from build123d import *

# Parameters (mm, degrees)
SKETCH_1_W          = 100
SKETCH_1_H          = 110
SKETCH_1_R          = 35
EXTRUDE_1_DEPTH     = 10
SKETCH_2_W          = 6
SKETCH_2_H          = 20
EXTRUDE_2_DEPTH     = 40
FILLET_1_R          = 20
FILLET_2_R          = 7
SKETCH_3_R          = 2.1
CUT_EXTRUDE_1_DEPTH = 111.01004512
FILLET_3_R          = 20


with BuildPart() as part:
    # 草图1 → 凸台-拉伸1 (new body)
    with BuildSketch(Plane.XY):
        Rectangle(SKETCH_1_W, SKETCH_1_H)
        Circle(SKETCH_1_R, mode=Mode.SUBTRACT)
    extrude(amount=EXTRUDE_1_DEPTH)

    # 草图2 → 凸台-拉伸2 (add)
    with BuildSketch(Plane.XY.offset(10)):
        with Locations((-28.1, 45)):
            Rectangle(SKETCH_2_W, SKETCH_2_H)
        with Locations((28.1, 45)):
            Rectangle(SKETCH_2_W, SKETCH_2_H)
        with Locations((28.1, -45)):
            Rectangle(SKETCH_2_W, SKETCH_2_H)
        with Locations((-28.1, -45)):
            Rectangle(SKETCH_2_W, SKETCH_2_H)
    extrude(amount=EXTRUDE_2_DEPTH)

    # 圆角1
    # the kernel refuses this fillet: 20 mm, written as the material it takes off along each edge
    with BuildSketch(Plane(origin=(0, 0, 0), x_dir=(1, 0, 0), z_dir=(0, -1, 0))) as fillet_1_piece_1:
        with BuildLine():
            CenterArc((52.320508076, 20), FILLET_1_R, 210, 60)
            Line((35, 10), (35, 0))
            Line((35, 0), (52.320508076, 0))
        make_face()
    revolve(axis=Axis((0, 0, 0), (0, 0, 1)), mode=Mode.SUBTRACT)

    # 圆角2
    fillet_2_edges = [part.edges().sort_by_distance(p)[0] for p in [
        (-31.1, 45, 10),
        (-28.1, 35, 10),
        (28.1, 35, 10),
        (31.1, 45, 10),
        (31.1, -45, 10),
        (28.1, -35, 10),
        (-28.1, -35, 10),
        (-31.1, -45, 10),
    ]]
    fillet(fillet_2_edges, radius=FILLET_2_R)

    # 草图3 → 切除-拉伸1 (cut, through all)
    with BuildSketch(Plane.ZY.offset(31.1)):
        with Locations(Location((20, -45, 0), (0, 0, 270))):
            Circle(SKETCH_3_R)
        with Locations(Location((40, -45, 0), (0, 0, 270))):
            Circle(SKETCH_3_R)
        with Locations(Location((40, 45, 0), (0, 0, 270))):
            Circle(SKETCH_3_R)
        with Locations(Location((20, 45, 0), (0, 0, 270))):
            Circle(SKETCH_3_R)
    extrude(amount=-CUT_EXTRUDE_1_DEPTH, mode=Mode.SUBTRACT)

    # 圆角3
    fillet_3_edges = [part.edges().sort_by_distance(p)[0] for p in [
        (50, -55, 5),
        (50, 55, 5),
        (-50, 55, 5),
        (-50, -55, 5),
    ]]
    fillet(fillet_3_edges, radius=FILLET_3_R)


solid = part.part
The model under review builds one solid part; all positions refer to its coordinate system, in mm. A direction names the side the tool comes from. Round coordinates to 2 decimals unless told otherwise and drop trailing zeros. Write each loop counter-clockwise with the first axis right and the second up, starting at its lowest first coordinate (ties: lowest second). Pieces come first, ordered by that corner, then holes. Notation, with made-up numbers: M -24.5,60.5 L 7.5,60.5 A6 ccw 7.5,64.5 Z; hole C -39.5,80 d11. An arc over 180 degrees is marked long. Answer as CSV lines item,"result". Start each with the question number.
Q1. Tool access review of faces 1 (the face through (-50, 0, 5)), 2 (the face through (28.06, -46.13, 21.77)), 3 (the face through (-25.1, -45, 30)), 4 (the face through (31.1, -45, 33)), 5 (the face through (30.25, -31.95, 11.22)): name each direction out of +Z, -Z, +X, -X, +Y, -Y from which nothing blocks a thin tool from reaching the whole face with its end or side.
Q2. Consider section A-A, the plane z = 34. Give the boundary of the cut face in (x, y).
Q3. Consider section C-C, the plane y = -45. State how many separate pieces and enclosed holes the cut face has, then the cut area to 3 significant figures.
Q4. Clearance check with flat-ended pins moving along their axes: P1, Ø5, axis at x = 17.5, y = 41, coming from the +Z side; P2, Ø5, axis at y = 45, z = 40, coming from the -X side; P3, Ø6, axis at x = 34.5, y = 7.5, coming from the -Z side. State where each tip first meets the part, or that it passes through.
Q5. Wall thickness on line 1 along Z through (x, y) = (29, -45); line 2 along Y through (x, z) = (-25.5, 32.5); line 3 along X through (y, z) = (-39, 44.5): over which ranges is each line inside the solid? List them lowest first.
Q6. Consider section B-B, the plane z = 7. Give the boundary of the cut face in (x, y).
Q7. The part is to be moulded in two halves that separate along Z. For faces 6 (the face through (28, 35, 33)), 7 (the face through (-28.14, 43.87, 21.77)), 8 (the face through (-33.2, -44.3, 12)), say which applies: +Z half, -Z half, draft (parallel to the pull), parting line (faces both ways), or undercut.
Result set:
1,face 1,"+Z, -Z, -X, +Y, -Y"
1,face 2,"+X, -X"
1,face 3,"+Z, +Y, -Y"
1,face 4,"+Z, +X, +Y, -Y"
1,face 5,"+Z, +X, -X"
2,outline,"M -31.1,-54.97 A20 ccw -30,-55 L -25.1,-55 L -25.1,-35 L -31.1,-35 Z; M -31.1,35 L -25.1,35 L -25.1,55 L -30,55 A20 ccw -31.1,54.97 Z; M 25.1,-55 L 30,-55 A20 ccw 31.1,-54.97 L 31.1,-35 L 25.1,-35 Z; M 25.1,35 L 31.1,35 L 31.1,54.97 A20 ccw 30,55 L 25.1,55 Z"
3,separate pieces,"5"
3,enclosed holes,"0"
3,area,"1,310 mm²"
4,P1,"stops at z = 10"
4,P2,"stops at x = -31.1"
4,P3,"stops at z = 5.73"
5,line 1,"z = 0 to 17.9, 22.1 to 37.9, 42.1 to 50"
5,line 2,"y = -55 to -35, 35 to 55"
5,line 3,"x = -31.1 to -25.1, 25.1 to 31.1"
6,outline,"M -50,-35 A20 ccw -30,-55 L 30,-55 A20 ccw 50,-35 L 50,35 A20 ccw 30,55 L -30,55 A20 ccw -50,35 Z; hole C 0,0 d74.24"
7,face 6,"draft"
7,face 7,"undercut"
7,face 8,"+Z half"
